```python
from build123d import *

# Parameters (mm, degrees)
CHAMFER1_SIZE = 0.878417015


with BuildPart() as part:
    # Sketch1 → Revolve1 (revolve)
    with BuildSketch(Plane(origin=(0, 0, 0), x_dir=(0, 0, -1), z_dir=(1, 0, 0))):
        with BuildLine():
            Line((0, 0), (0, 10))
            ThreePointArc((0, 10), (10, 0), (0, -10))
            Line((0, -10), (0, 0))
        make_face()
    revolve(axis=Axis((0, 0, 0), (0, 1, 0)))

    # Sketch2 → Cut-Revolve1 (revolve, cut)
    with BuildSketch(Plane(origin=(0, 0, 0), x_dir=(0, 0, -1), z_dir=(1, 0, 0)), mode=Mode.PRIVATE) as cut_revolve1_sk:
        Polygon((0, 0), (0, 10.64), (2.2, 10.64), (1.5, 0), align=None)
    revolve(cut_revolve1_sk.sketch.rotate(Axis((0, 0, 0), (0, 1, 0)), 180), axis=Axis((0, 0, 0), (0, 1, 0)), mode=Mode.SUBTRACT)

    # Chamfer1
    # the kernel refuses this chamfer: 1, 0.878417015 mm, written as the material it takes off along each edge
    with BuildSketch(Plane(origin=(0, 9.767763137, 0), x_dir=(0, 0, 1), z_dir=(-1, 0, 0))) as chamfer1_piece_1:
        with BuildLine():
            Line((3.065028643, -0.249065777), (2.142615996 - CHAMFER1_SIZE * 0.0656475573893, -CHAMFER1_SIZE * 0.997842872317))
            Line((2.142615996 - CHAMFER1_SIZE * 0.0656475573893, -CHAMFER1_SIZE * 0.997842872317), (2.142615996, 0))
            ThreePointArc((2.142615996, 0), (2.619777215, -0.117023924), (3.065028643, -0.249065777))
        make_face()
    revolve(axis=Axis((0, 9.767763137, 0), (0, 1, 0)), revolution_arc=180, mode=Mode.SUBTRACT)
    with BuildSketch(Plane(origin=(0, 9.767763137, 0), x_dir=(0, 0, -1), z_dir=(1, 0, 0))) as chamfer1_piece_2:
        with BuildLine():
            Line((3.065028643, -0.249065777), (2.142615996 - CHAMFER1_SIZE * 0.0656475573893, -CHAMFER1_SIZE * 0.997842872317))
            Line((2.142615996 - CHAMFER1_SIZE * 0.0656475573893, -CHAMFER1_SIZE * 0.997842872317), (2.142615996, 0))
            ThreePointArc((2.142615996, 0), (2.619777215, -0.117023924), (3.065028643, -0.249065777))
        make_face()
    revolve(axis=Axis((0, 9.767763137, 0), (0, 1, 0)), revolution_arc=180, mode=Mode.SUBTRACT)


solid = part.part
```
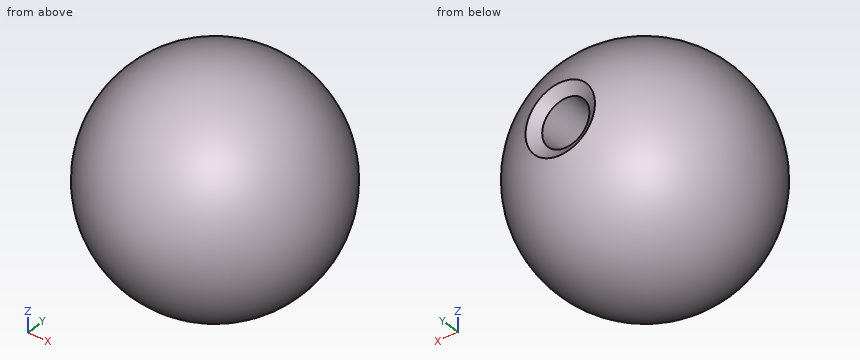
Part model, mm, in its own coordinate system. Coordinates: 2 decimals unless noted, no trailing zeros. Write each loop counter-clockwise with the first axis right and the second up, starting at its lowest first coordinate (ties: lowest second). Pieces come first, ordered by that corner, then holes.
Item 1: Slice it at A-A (z = 0). Write the cut outline in (x, y), and give its area (3 significant figures).
Item 2: Slice it at B-B (y = -8). Write the cut outline in (x, z).
Item 3: Slice it at D-D (y = 6.75). Write the cut outline in (x, z), and give its area (3 significant figures).
Item 4: Probe line 1 (Z direction, x = -1.25, y = 0.5); line 2 (Z direction, x = 0, y = 2.5); line 3 (X direction, y = 8.5, z = -0.25). List the from-to ranges inside material, lowest first.
Item 5: Slice it at C-C (x = 0). Write the cut outline in (y, z).
Item 6: Pin check, flat tips, straight feed: pin 1 (1.5 mm diameter, centred on x = -3, z = -5.5, fed in from -Y); pin 2 (1 mm diameter, centred on y = 3, z = 0.5, fed in from +X); pin 3 (4 mm diameter, centred on y = 0, z = 5.5, fed in from +X). Stop position of each tip, or through.
Results found:
1. outline: (-3.07, 9.52) arc R10 ccw (long way) to (3.07, 9.52) - (2.08, 8.89) - (1.5, 0) - (-1.5, 0) - (-2.08, 8.89) - close
1. area: 277 mm2
2. outline: circle Ø12 at (0, 0)
3. outline: circle Ø14.76 at (0, 0); hole circle Ø3.89 at (0, 0)
3. area: 159 mm2
4. line 1: z = -9.91 to -0.89, 0.89 to 9.91
4. line 2: z = -9.68 to -1.66, 1.66 to 9.68
4. line 3: x = -5.26 to -2.04, 2.04 to 5.26
5. outline: (0, -1.5) - (0, 1.5) - (8.89, 2.08) - (9.52, 3.07) arc R10 ccw (long way) to (9.52, -3.07) - (8.89, -2.08) - close
6. pin 1: stops at y = -8.34
6. pin 2: stops at x = 9.67
6. pin 3: stops at x = 9.37
